Autodesk Inventor part; units mm, degrees
ref_plane "Work Plane1" through (12.5, 0, 0) normal (1, 0, 0) x (0, 1, 0)
ref_plane "XZ Plane" through (0, 0, 0) normal (0, 1, 0) x (-1, 0, 0)
ref_plane "XY Plane" through (0, 0, 0) normal (0, 0, 1) x (1, 0, 0)
sketch "Sketch1" plane through (0, 0, 0) normal (0, 0, 1) x (1, 0, 0)
  line L0 (-12.5, -20) -> (-12.5, 20)
  arc A0 (12.5, 20) -> (-12.5, 20) centre (0, 20) ccw
  arc A1 (-12.5, -20) -> (12.5, -20) centre (0, -20) ccw
  line L1 (12.5, -20) -> (12.5, 20)
  arc A2 (6.25, 20) -> (-6.25, 20) centre (0, 20) ccw
  arc A3 (-6.25, -20) -> (6.25, -20) centre (0, -20) ccw
  line L2 (6.25, -20) -> (6.25, 20)
  line L3 (-6.25, -20) -> (-6.25, 20)
  point P0 (0, 0)
  point P1 (12.5, 0)
  dimension "d0" = 40
  dimension "d1" = 12.5
  dimension "d2" = 12.5
extrude "Extrusion1" add sketch "Sketch1" along normal mid plane 28
ref_plane "Work Plane1" through (12.5, 0, 0) normal (1, 0, 0) x (0, 1, 0)
sketch "Sketch2" plane through (12.5, 0, 0) normal (1, 0, 0) x (0, 1, 0)
  line L0 (20, 14) -> (20, -14) construction
  line L1 (-20, 14) -> (20, 14) construction
  line L2 (-20, -14) -> (-20, 14) construction
  line L3 (20, -14) -> (-20, -14) construction
  circle A0 centre (19, 0) radius 4.3
  line L4 (0, 14) -> (0, -14) construction
  line L5 (-20, -14) -> (20, -14) construction
  circle A1 centre (-19, 0) radius 4.3
  point P0 (0, 0)
  point P1 (20, 0)
  dimension "d6" = 8.6
  dimension "d10" = 38
extrude "Extrusion2" cut sketch "Sketch2" against normal blind 28
properties part number "cabeza_obj2"
Here's how the part is built. I have some questions about the finished solid (model axes, mm). A direction names the side the tool comes from. Coordinates: 2 decimals unless noted, no trailing zeros. Write each loop counter-clockwise with the first axis right and the second up, starting at its lowest first coordinate (ties: lowest second). Pieces come first, ordered by that corner, then holes.
1) If we section it at A-A (y = -19): List the corners of the cut face in (x, z) for me, plus the area to 4 significant figures.
Filled in:
outline: (-12.5, -14) - (-6.25, -14) - (-6.25, -4.3) - (-12.5, -4.3) - close; (-12.5, 4.3) - (-6.25, 4.3) - (-6.25, 14) - (-12.5, 14) - close; (6.25, -14) - (12.5, -14) - (12.5, -4.3) - (6.25, -4.3) - close; (6.25, 4.3) - (12.5, 4.3) - (12.5, 14) - (6.25, 14) - close
area: 242.5 mm2
2) Thinking about a two-plate mould opening in Z: for faces 3 (the face through (8.954, -17.016, -3.815)), 4 (the face through (-6.25, 0, 0)), 5 (the face through (-8.853, -23.296, 0.189)), 6 (the face through (8, 0, 14)), which applies, +Z half, -Z half, draft (parallel to the pull), parting line (faces both ways), or undercut?
Filled in:
face 3: undercut
face 4: draft
face 5: undercut
face 6: +Z half
3) Which directions (+Z, -Z, +X, -X, +Y, -Y) give clear straight access to the entire face, cutting with the end or side of a thin tool? Please do faces 1 (the face through (-12.5, 0, 0)), 2 (the face through (-0.14, 26.25, -0.2)).
Filled in:
face 1: +Z, -Z, -X, +Y, -Y
face 2: +Z, -Z
4) If we section it at D-D (x = -3.75): List the corners of the cut face in (y, z) for me, plus the area to 3 significant figures.
Filled in:
outline: (-31.92, -14) - (-25, -14) - (-25, 14) - (-31.92, 14) - close; (25, -14) - (31.92, -14) - (31.92, 14) - (25, 14) - close
area: 388 mm2
5) If I drill on line 1 (X direction, y = 14.5, z = 3); line 2 (Z direction, x = -7, y = 19); line 3 (Y direction, x = -7.75, z = 0), over which ranges is the centre line in solid material (lowest first)?
Filled in:
line 1: x = -12.5 to -6.25, 6.25 to 12.5
line 2: z = -14 to -4.3, 4.3 to 14
line 3: y = -29.81 to -23.3, -14.7 to 14.7, 23.3 to 29.81
6) If we section it at C-C (y = 12.5): List the corners of the cut face in (x, z) for me.
Filled in:
outline: (-12.5, -14) - (-6.25, -14) - (-6.25, 14) - (-12.5, 14) - close; (6.25, -14) - (12.5, -14) - (12.5, 14) - (6.25, 14) - close
7) If we section it at B-B (z = -6.75): List the corners of the cut face in (x, y) for me.
Filled in:
outline: (-12.5, -20) arc R12.5 ccw to (12.5, -20) - (12.5, 20) arc R12.5 ccw to (-12.5, 20) - close; hole (-6.25, -20) arc R6.25 ccw to (6.25, -20) - (6.25, 20) arc R6.25 ccw to (-6.25, 20) - close
8) I'm going to push flat-ended pins straight in: pin 1 (8 mm diameter, centred on y = -25.5, z = -9, fed in from +X); pin 2 (2 mm diameter, centred on x = 4, y = 15.5, fed in from -Z) (1 decimal); pin 3 (3 mm diameter, centred on y = 26, z = 7.5, fed in from -X); pin 4 (6 mm diameter, centred on x = 5, z = 1, fed in from -Y). Where does each tip first touch, or does it pass through?
Filled in:
pin 1: stops at x = 12.41
pin 2: passes through
pin 3: stops at x = -11.66
pin 4: stops at y = -32.34
